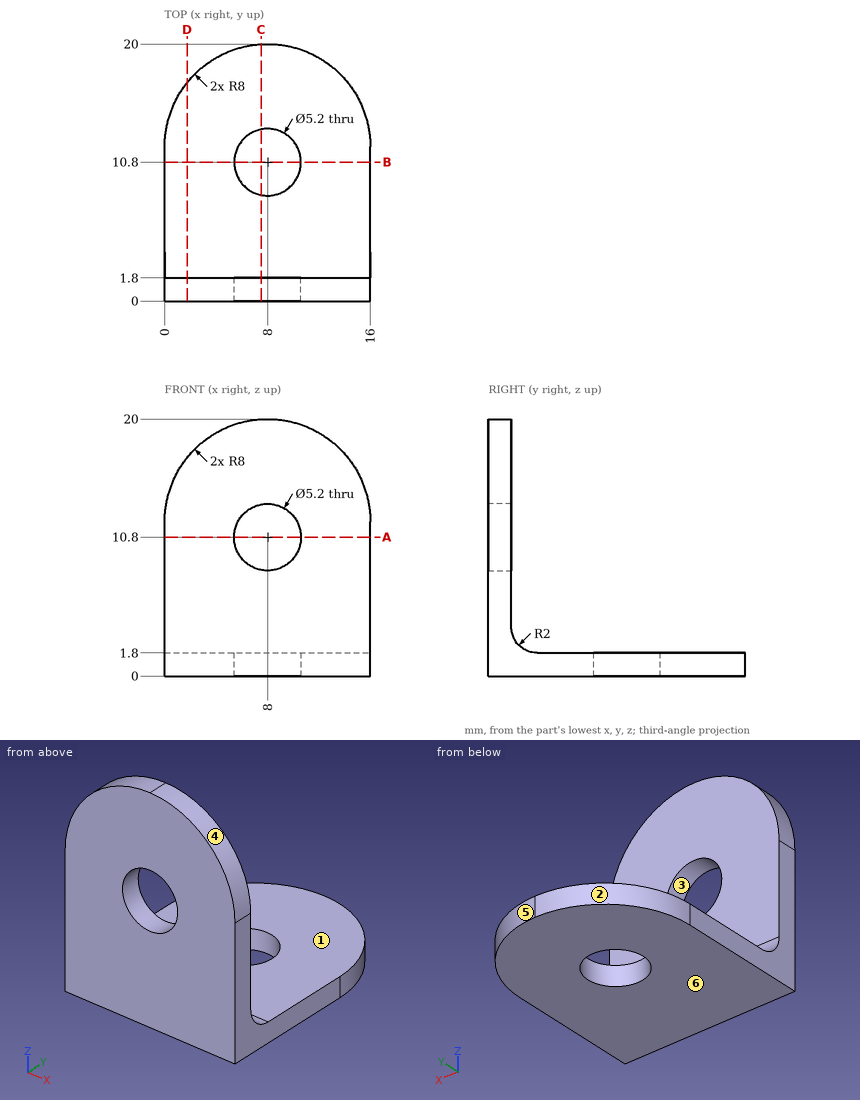
Geometry check sheet. Reference: drawing and pictorial views, mm from the part's lowest x, y, z. A direction names the side the tool comes from. Coordinates: 2 decimals unless noted, no trailing zeros. Order: outer loops, then holes, each group sorted by start corner. A loop starts at its lowest first (then second) coordinate and runs counter-clockwise, first axis right, second up.
1. Sectioned sample at C-C, the plane x = 7.5. Record the cut outline in (y, z), and give its area (3 significant figures).
Results found:
outline: (0, 0) - (8.25, 0) - (8.25, 1.8) - (3.8, 1.8) arc R2 cw to (1.8, 3.8) - (1.8, 8.25) - (0, 8.25) - close; (0, 13.35) - (1.8, 13.35) - (1.8, 19.98) - (0, 19.98) - close; (13.35, 0) - (19.98, 0) - (19.98, 1.8) - (13.35, 1.8) - close
area: 51.2 mm2
2. Scan lines: line 1 (X direction, y = 0.9, z = 10.8); line 2 (Y direction, x = 8, z = 0.8); line 3 (Y direction, x = 13, z = 15.25). Record each from-to range of solid material in increasing order.
Results found:
line 1: x = 0 to 5.4, 10.6 to 16
line 2: y = 0 to 8.2, 13.4 to 20
line 3: y = 0 to 1.8
3. Sectioned sample at D-D, the plane x = 1.75. Record the cut outline in (y, z), and give its area (3 significant figures).
Results found:
outline: (0, 0) - (16.99, 0) - (16.99, 1.8) - (3.8, 1.8) arc R2 cw to (1.8, 3.8) - (1.8, 16.99) - (0, 16.99) - close
area: 58.8 mm2
4. Set-up check for the marked faces 1 and 2: record each of +Z, -Z, +X, -X, +Y, -Y from which the full face is reachable in a straight line by a thin tool's end or side.
Results found:
face 1: +Z, +X, -X, +Y
face 2: +Z, -Z, -X, +Y
5. Sectioned sample at A-A, the plane z = 10.8. Record the cut outline in (x, y).
Results found:
outline: (0, 0) - (5.4, 0) - (5.4, 1.8) - (0, 1.8) - close; (10.6, 0) - (16, 0) - (16, 1.8) - (10.6, 1.8) - close
6. Go/stop test with flat-tipped pins: pin 1 Ø8 at (x, y) = (9, 12) entering from +Z; pin 2 Ø8 at (x, z) = (8, 13.5) entering from -Y; pin 3 Ø2 at (x, y) = (14, 4) entering from +Z; pin 4 Ø4 at (x, z) = (10, 6) entering from +Y. Record where each tip stops, or that it passes through.
Results found:
pin 1: stops at z = 1.8
pin 2: stops at y = 0
pin 3: stops at z = 1.97
pin 4: stops at y = 1.8
7. Release check for a two-part mould opening along Z. For the marked faces 3, 4, 5 and 6 record: +Z half, -Z half, draft (parallel to the pull), parting line (faces both ways), or undercut.
Results found:
face 3: undercut
face 4: +Z half
face 5: draft
face 6: -Z half
